```python
from build123d import *

# Parameters (mm, degrees)
BOSS_EXTRUDE1_DEPTH = 100
BOSS_EXTRUDE2_DEPTH = 12.5
BOSS_EXTRUDE3_REACH = 116.264
SKETCH7_W           = 5
SKETCH7_H           = 10


with BuildPart() as part:
    # Sketch3 → Boss-Extrude1 (new body)
    with BuildSketch(Plane.XY):
        Polygon((11.547005384, 0), (5.773502692, 10), (-5.773502692, 10), (-11.547005384, 0), (-5.773502692, -10), (5.773502692, -10), align=None)
        Polygon((5.773502692, 0), (2.886751346, 5), (-2.886751346, 5), (-5.773502692, 0), (-2.886751346, -5), (2.886751346, -5), align=None, mode=Mode.SUBTRACT)
    extrude(amount=BOSS_EXTRUDE1_DEPTH)

    # Sketch5 → Boss-Extrude2 (add)
    with BuildSketch(Plane.XY.offset(100)):
        Polygon((5.773502692, 5), (8.660254038, 5), (11.547005384, 0), (8.660254038, -5), (5.773502692, -5), align=None)
        Polygon((-8.660254038, 5), (-11.547005384, 0), (-8.660254038, -5), (-5.773502692, -5), (-5.773502692, 5), align=None)
    boss_extrude2 = extrude(amount=BOSS_EXTRUDE2_DEPTH)

    # Sketch7 → Boss-Extrude3 (add, up to next)
    with BuildSketch(Plane(origin=(-5.773502692, 0, 0), x_dir=(0, 0, -1), z_dir=(1, 0, 0)), mode=Mode.PRIVATE) as boss_extrude3_sk1:
        with Locations((-110, 0)):
            Rectangle(SKETCH7_W, SKETCH7_H)
    boss_extrude3_tool1 = extrude(boss_extrude3_sk1.sketch, amount=BOSS_EXTRUDE3_REACH, mode=Mode.PRIVATE) - part.part
    boss_extrude3 = boss_extrude3_tool1.solids().sort_by_distance((-5.773503, 0, 110))[0]
    add(boss_extrude3)

    # Mirror1: Boss-Extrude2, Boss-Extrude3 across plane
    add(boss_extrude2.mirror(Plane.XY.offset(50)))
    add(boss_extrude3.mirror(Plane.XY.offset(50)))


solid = part.part
```
Can you work these out from the model? Positions are in its coordinate system, mm. A direction names the side the tool comes from. Coordinates: 2 decimals unless noted, no trailing zeros. Order: outer loops, then holes, each group sorted by start corner. A loop starts at its lowest first (then second) coordinate and runs counter-clockwise, first axis right, second up.
1. If we section it at C-C (x = -4.5): Please give me the cut outline in (y, z).
2. I need wall thicknesses on line 1 (Z direction, x = -5.5, y = -4.75); line 2 (Y direction, x = -1.75, z = 33.5); line 3 (Z direction, x = -0.75, y = 2.5). Which ranges of each line are inside material? Lowest first, please.
3. Thinking about a two-plate mould opening in Y: for faces 4 (the face through (0, 5, 108)), 5 (the face through (0, 5, 49)), 6 (the face through (0, -5, -8)), which applies, +Y half, -Y half, draft (parallel to the pull), parting line (faces both ways), or undercut?
4. For faces 1 (the face through (0, -7, 0)), 2 (the face through (5.774, 0, 104)), 3 (the face through (0, -5, 108)), which set-ups out of +Z, -Z, +X, -X, +Y, -Y let a thin tool reach every point of the face, with its end or its side?
5. If we section it at A-A (z = 40): Please give me the cut outline in (x, y).
6. If we section it at B-B (y = 3.75): Please give me the cut outline in (x, z).
7. I'm going to push flat-ended pins straight in: pin 1 (2 mm diameter, centred on y = 0.5, z = -2.5, fed in from +X); pin 2 (1.5 mm diameter, centred on y = 1, z = 78, fed in from +X); pin 3 (6 mm diameter, centred on y = -7, z = 19.5, fed in from +X). Where does each tip first touch, or does it pass through?
8. If we section it at D-D (x = 7.5): Please give me the cut outline in (y, z), then the cut area to 3 significant figures.
Entries:
1. outline: (-10, 0) - (-2.21, 0) - (-2.21, 100) - (-10, 100) - close; (-5, -12.5) - (5, -12.5) - (5, -7.5) - (-5, -7.5) - close; (-5, 107.5) - (5, 107.5) - (5, 112.5) - (-5, 112.5) - close; (2.21, 0) - (10, 0) - (10, 100) - (2.21, 100) - close
2. line 1: z = -12.5 to -7.5, 0 to 100, 107.5 to 112.5
2. line 2: y = -10 to -5, 5 to 10
2. line 3: z = -12.5 to -7.5, 107.5 to 112.5
3. face 4: +Y half
3. face 5: undercut
3. face 6: -Y half
4. face 1: -Y
4. face 2: +Y, -Y
4. face 3: +Z, +X, -X, -Y
5. outline: (-11.55, 0) - (-5.77, -10) - (5.77, -10) - (11.55, 0) - (5.77, 10) - (-5.77, 10) - close; hole (-5.77, 0) - (-2.89, -5) - (2.89, -5) - (5.77, 0) - (2.89, 5) - (-2.89, 5) - close
6. outline: (-9.38, -12.5) - (9.38, -12.5) - (9.38, 112.5) - (-9.38, 112.5) - close; hole (-5.77, -7.5) - (5.77, -7.5) - (5.77, 0) - (3.61, 0) - (3.61, 100) - (5.77, 100) - (5.77, 107.5) - (-5.77, 107.5) - (-5.77, 100) - (-3.61, 100) - (-3.61, 0) - (-5.77, 0) - close
7. pin 1: stops at x = 11.55
7. pin 2: stops at x = 11.4
7. pin 3: stops at x = 9.24
8. outline: (-7.01, 0) - (-5, 0) - (-5, -12.5) - (5, -12.5) - (5, 0) - (7.01, 0) - (7.01, 100) - (5, 100) - (5, 112.5) - (-5, 112.5) - (-5, 100) - (-7.01, 100) - close
8. area: 1,650 mm2
